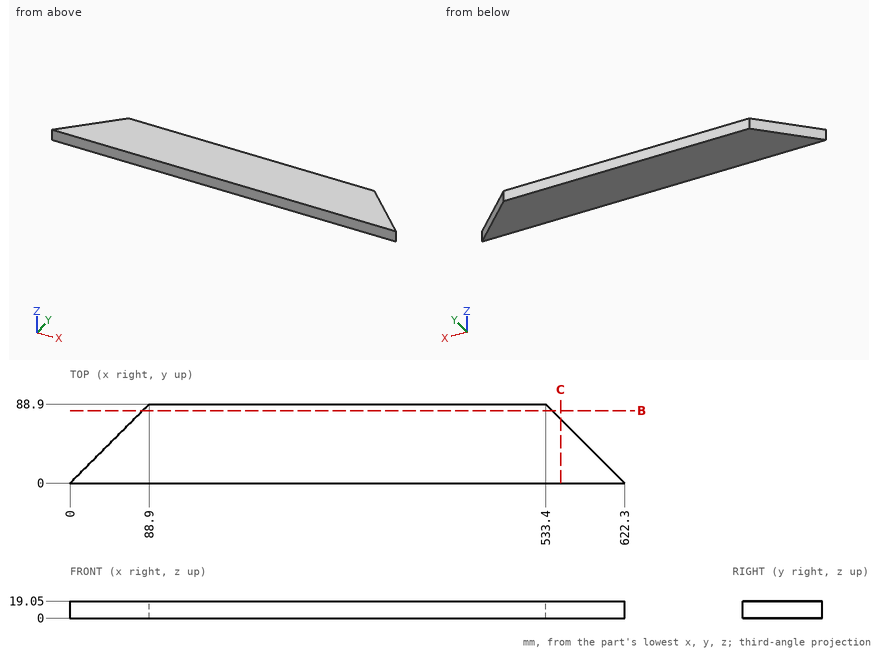
Design review of the part shown in the three views and the two pictorial views. Dimensions are in mm from the part's minimum x, y and z. Round coordinates to 2 decimals unless told otherwise and drop trailing zeros. Order: outer loops, then holes, each group sorted by start corner. A loop starts at its lowest first (then second) coordinate and runs counter-clockwise, first axis right, second up. Notation, with made-up numbers: (7, 65) - (46, 65) arc R29 ccw to (46, 92) - close; hole circle Ø8 at (8.25, -37). An arc over 180 degrees is marked (long way). Answer in a Markdown table with one row per item.
(1) For line 1 (X direction, y = 9, z = 1.75); line 2 (X direction, y = 74, z = 7.75); line 3 (Y direction, x = 596.5, z = 2.75), list the stretches that pass through material, from the lowest coordinate up. Write a range as from..to.
Result set:
| item | result |
|---|---|
| line 1 | x = 9..613.3 |
| line 2 | x = 74..548.3 |
| line 3 | y = 0..25.8 |
(2) Take a section at B-B on y = 81.5. Write out the cut boundary in (x, z), plus the area to 3 significant figures.
Result set:
| item | result |
|---|---|
| outline | (81.5, 0) - (540.8, 0) - (540.8, 19.05) - (81.5, 19.05) - close |
| area | 8,750 mm2 |
(3) Clearance check with flat-ended pins moving along their axes: P1, Ø12, axis at x = 66, y = 58, coming from the -Z side; P2, Ø5, axis at y = 76.5, z = 12, coming from the +X side; P3, Ø10, axis at y = 44.5, z = 12.5, coming from the -X side. State where each tip first meets the part, or that it passes through.
Result set:
| item | result |
|---|---|
| P1 | stops at z = 0 |
| P2 | stops at x = 548.3 |
| P3 | stops at x = 39.5 |
(4) Take a section at C-C on x = 550.5. Write out the cut boundary in (y, z).
Result set:
| item | result |
|---|---|
| outline | (0, 0) - (71.8, 0) - (71.8, 19.05) - (0, 19.05) - close |
